Autodesk Inventor part; units mm, degrees
ref_plane "YZ Plane" through (0, 0, 0) normal (1, 0, 0) x (0, 1, 0)
ref_plane "XZ Plane" through (0, 0, 0) normal (0, 1, 0) x (-1, 0, 0)
ref_plane "XY Plane" through (0, 0, 0) normal (0, 0, 1) x (1, 0, 0)
sketch "Skizze1" plane through (0, 0, 0) normal (0, 0, 1) x (1, 0, 0)
  line L0 (0, 0) -> (-40.8899, -4.2977)
  line L1 (-40.8899, -4.2977) -> (-40.8899, -33.7977)
  line L2 (-40.8899, -33.7977) -> (-0.5899, -33.7977)
  line L3 (-0.5899, -33.7977) -> (0, 0)
  line L4 (-43.8899, -0.591) -> (3.0763, 4.3454)
  line L5 (-43.8899, -36.7977) -> (-43.8899, -0.591)
  line L6 (-43.8899, -36.7977) -> (2.3582, -36.7977)
  line L7 (2.3582, -36.7977) -> (3.0763, 4.3454)
  dimension "d1" = 29.5
  dimension "d2" = 40.3
  dimension "d6" = 90
  dimension "d9" = 91
  dimension "d12" = 96
  dimension "d13" = 41.1152
  dimension "d14" = 33.8028
  dimension "d22" = 4
  dimension "d23" = 3
  dimension "d24" = 3
  dimension "d25" = 3
extrude "Extrusion1" add sketch "Skizze1" along normal blind 57
sketch "Skizze3" plane through (-43.8899, -36.7977, 0) normal (0, -1, 0) x (1, 0, 0)
  line L0 (0, 0) -> (46.2481, 0) construction
  line L1 (46.2481, 0) -> (46.2481, 57) construction
  line L2 (0, 57) -> (46.2481, 57) construction
  line L3 (0, 0) -> (0, 57)
  line L4 (0, 0) -> (46.2481, 0)
  line L5 (0, 57) -> (46.2481, 57)
  line L6 (0, 57) -> (46.9662, 45.29)
  line L7 (46.2481, 0) -> (46.2481, 57)
  line L8 (46.2481, 0) -> (46.9662, 0)
  line L9 (46.2481, 0) -> (46.9662, 0)
  line L10 (46.9662, 0) -> (46.9662, 2.4614)
  line L11 (46.9662, 2.4614) -> (0, 0)
  line L12 (46.9662, 0) -> (46.9662, 57)
  line L13 (46.9662, 45.29) -> (46.9662, 57)
  line L14 (46.9662, 57) -> (46.9662, 57)
  line L15 (0, 57) -> (46.9662, 57)
  point P0 (43.8899, 0)
  dimension "d27" = 76
  dimension "d30" = 87
extrude "Extrusion3" cut sketch "Skizze3" against normal blind 57 contours L11 L7 L4 | L5 L7 L6 | L7 L11 L10 L8 | L15 L12 L6 L7
fillet "Rundung1" radius 3 4 edges at (-43.8899, -36.7977, 28.5) (-43.8899, -0.591, 28.5) (2.3582, -36.7977, 23.9464) (3.0763, 4.3454, 23.8757)
equation "\"d24\" = d23"
equation "\"d25\" = d24"
properties part number "handle_top_final"
Work out the finished part from the listing and answer in its coordinate system (mm). A direction names the side the tool comes from. Give positions to 0.01 mm unless a question says otherwise; leave off trailing zeros. Loops run counter-clockwise (first coordinate to the right, second up) from the corner with the lowest first, then second, coordinate; pieces in that order, holes last. Notation, with made-up numbers: (-23, 68) -> (20, 68) arc R16 ccw to (20, 79) -> close; hole circle Ø5 at (60, 88.5). An arc over 180 degrees is marked (long way). Write item = value, one per line. Start each with the question number.
(1) Find the intervals of material crossed by probe 1 along X at (y, z) = (-19, 50); probe 2 along Y at (x, z) = (-12, 5); probe 3 along Y at (x, z) = (-38, 25), in increasing order. Write a range as from..to.
(2) Find section A-A on y = -12.5. Give the vertices of the cut face in (x, z), and give its area (3 significant figures).
(3) Which of the six approach directions +Z, -Z, +X, -X, +Y, -Y give full straight-line access (tool end or side, diameter ignored) to faces 4 (the flat face through (-20.765, -34.816, 51.234)), 5 (the flat face through (-40.89, -19, 28))?
(4) Find section C-C on x = -37. Give the vertices of the cut face in (y, z), and give its area (3 significant figures).
(5) Given pin 1 Ø4 at (y, z) = (-3, 19) entering from -X; pin 2 Ø4 at (x, z) = (-26, 47) entering from +Y; pin 3 Ø6 at (y, z) = (-18, 43) entering from +X; pin 4 Ø8 at (y, z) = (-25, 43) entering from +X, each flat-ended and moving along its own axis, determine where each tip first touches the part or whether it passes through.
(6) Find section B-B on z = 17. Give the vertices of the cut face in (x, y).
(7) The mould has two halves that part along X. Classify faces 1 (the flat face through (-20.16, -2.12, 27.81)), 2 (the flat face through (-20.108, -34.816, 1.246)), 3 (the cylindrical face through (-43.03, -35.9, 28.9)): +X half, -X half, draft (parallel to the pull), parting line (faces both ways), or undercut.
From the geometry:
q1.probe_1 = -43.89..-40.89
q1.probe_2 = -36.8..-33.8, -1.26..2.76
q1.probe_3 = -36.8..-33.8, -3.99..0.03
q2.outline = (-43.89, 0) -> (-40.89, 0.16) -> (-40.89, 56.25) -> (-43.89, 57) -> close; (-0.22, 2.29) -> (2.78, 2.45) -> (2.78, 45.36) -> (-0.22, 46.11) -> close
q2.area = 300 mm^2
q3.face_4 = +Z, +X, +Y, -Y
q3.face_5 = +Z, -Z
q4.outline = (-36.8, 0.36) -> (-33.8, 0.36) -> (-33.8, 55.28) -> (-36.8, 55.28) -> close; (-3.89, 0.36) -> (0.13, 0.36) -> (0.13, 55.28) -> (-3.89, 55.28) -> close
q4.area = 386 mm^2
q5.pin_1 = -43.89
q5.pin_2 = 1.5
q5.pin_3 = 2.74
q5.pin_4 = 2.63
q6.outline = (-43.89, -33.8) arc R3 ccw to (-40.89, -36.8) -> (-0.59, -36.8) arc R3 ccw to (2.41, -33.85) -> (3.02, 0.96) arc R3 ccw to (-0.3, 3.99) -> (-41.2, -0.31) arc R3 ccw to (-43.89, -3.29) -> close; hole (-40.89, -33.8) -> (-0.59, -33.8) -> (0, 0) -> (-40.89, -4.3) -> close
q7.face_1 = undercut
q7.face_2 = +X half
q7.face_3 = -X half
